Geometry: final body of the model. Coordinates: model frame, mm. A direction names the side the tool comes from. Give positions to 0.01 mm unless a question says otherwise; leave off trailing zeros. Write each loop counter-clockwise with the first axis right and the second up, starting at its lowest first coordinate (ties: lowest second). Pieces come first, ordered by that corner, then holes. Notation, with made-up numbers: (47.25, 81.5) - (99.25, 81.5) arc R21 cw to (99.25, 94.5) - close; hole circle Ø1 at (3.5, 61.5). An arc over 180 degrees is marked (long way). Return JSON: item names as keys, results as strings.
from build123d import *

# Parameters (mm, degrees)
SCHIZZO1_R                   = 1.75
ESTRUSIONE_ESTRUSIONE1_DEPTH = 3


with BuildPart() as part:
    # Schizzo1 → Estrusione-Estrusione1 (new body)
    with BuildSketch(Plane.XY):
        with BuildLine():
            Line((-5.892848523, 55.177208486), (-5.574209769, 52.193660395))
            Line((-5.574209769, 52.193660395), (-5.469026549, 51.208785854))
            ThreePointArc((-5.469026549, 51.208785854), (-8.668981909, 46.543993716), (-13.333774047, 49.743949076))
            Line((-13.333774047, 49.743949076), (-13.590216265, 50.700651099))
            ThreePointArc((-13.590216265, 50.700651099), (-14.064469506, 51.31253651), (-14.833377583, 51.402537967))
            ThreePointArc((-14.833377583, 51.402537967), (0, -53.5), (14.833377583, 51.402537967))
            ThreePointArc((14.833377583, 51.402537967), (14.064469506, 51.31253651), (13.590216265, 50.700651099))
            Line((13.590216265, 50.700651099), (13.333774047, 49.743949076))
            ThreePointArc((13.333774047, 49.743949076), (8.668981909, 46.543993716), (5.469026549, 51.208785854))
            Line((5.469026549, 51.208785854), (5.574209769, 52.193660395))
            Line((5.574209769, 52.193660395), (5.892848523, 55.177208486))
            ThreePointArc((5.892848523, 55.177208486), (6.266213098, 55.854839586), (7.011287463, 56.063284314))
            ThreePointArc((7.011287463, 56.063284314), (0, -56.5), (-7.011287463, 56.063284314))
            ThreePointArc((-7.011287463, 56.063284314), (-6.266213098, 55.854839586), (-5.892848523, 55.177208486))
        make_face()
        with Locations((-9.401400298, 50.476367465)):
            Circle(SCHIZZO1_R, mode=Mode.SUBTRACT)
        with Locations((9.401400298, 50.476367465)):
            Circle(SCHIZZO1_R, mode=Mode.SUBTRACT)
    extrude(amount=ESTRUSIONE_ESTRUSIONE1_DEPTH)


solid = part.part
Q1. Pin query (flat end, axial travel): P1, Ø1, axis at x = -39.5, z = 0.5, coming from the +Y side. Return the tip coordinate at first contact, or that it passes through.
Answer key:
{"P1": "stops at y = 40.88"}
Q2. Section query A-A, the plane y = 0. Return the cut outline in (x, z), plus the area to 3 significant figures.
Answer key:
{"outline": "(-56.5, 0) - (-53.5, 0) - (-53.5, 3) - (-56.5, 3) - close; (53.5, 0) - (56.5, 0) - (56.5, 3) - (53.5, 3) - close", "area": "18.0 mm^2"}
Q3. Section query B-B, the plane x = -24.5. Return the cut outline in (y, z).
Answer key:
{"outline": "(-50.91, 0) - (-47.56, 0) - (-47.56, 3) - (-50.91, 3) - close; (47.56, 0) - (50.91, 0) - (50.91, 3) - (47.56, 3) - close"}
Q4. Mould query, pull axis Y, two halves, no side actions, for faces 1 (the cylindrical face through (-8.46, 51.95, 1.48)), 2 (the cylindrical face through (2.39, -56.45, 1.48)), 3 (the flat face through (42.1, -33.3, 3)). Classes: pulls with the +Y half, pulls with the -Y half, needs draft (parallel to the pull), parting line crosses it, or undercut.
Answer key:
{"face 1": "undercut", "face 2": "parting line crosses it", "face 3": "needs draft"}
Q5. Material intervals for probe 1 along X at (y, z) = (16, 0.8); probe 2 along Y at (x, z) = (39, 0.95); probe 3 along X at (y, z) = (-27, 0.9), sorted ascending. Write a range as [from, to].
Answer key:
{"probe 1": "x = [-54.19, -51.05], [51.05, 54.19]", "probe 2": "y = [-40.88, -36.62], [36.62, 40.88]", "probe 3": "x = [-49.63, -46.19], [46.19, 49.63]"}
Q6. Section query D-D, the plane x = 0. Return the cut outline in (y, z).
Answer key:
{"outline": "(-56.5, 0) - (-53.5, 0) - (-53.5, 3) - (-56.5, 3) - close"}
Q7. Set-up query: faces 4 (the cylindrical face through (8.76, 46.53, 1.48)), 5 (the flat face through (42.1, -33.3, 0)). Return all of +Z, -Z, +X, -X, +Y, -Y with unobstructed straight access to the full face (end or side cutting, diameter ignored); none if empty.
Answer key:
{"face 4": "+Z, -Z", "face 5": "-Z, +X, -X, +Y, -Y"}
Q8. Section query C-C, the plane z = 1.25. Return the cut outline in (x, y).
Answer key:
{"outline": "(-14.83, 51.4) arc R1 cw to (-13.59, 50.7) - (-13.33, 49.74) arc R4 ccw to (-5.47, 51.21) - (-5.89, 55.18) arc R1 ccw to (-7.01, 56.06) arc R56.5 ccw (long way) to (7.01, 56.06) arc R1 ccw to (5.89, 55.18) - (5.47, 51.21) arc R4 ccw to (13.33, 49.74) - (13.59, 50.7) arc R1 cw to (14.83, 51.4) arc R53.5 cw (long way) to start; hole circle Ø3.5 at (-9.4, 50.48); hole circle Ø3.5 at (9.4, 50.48)"}
